Part print with two shaded views. Sizes in mm from the minimum x, y, z corner. A direction names the side the tool comes from. Round coordinates to 2 decimals unless told otherwise and drop trailing zeros. Order: outer loops, then holes, each group sorted by start corner. A loop starts at its lowest first (then second) coordinate and runs counter-clockwise, first axis right, second up. Notation, with made-up numbers: M 9,49.5 L 40,49.5 A28 cw 40,74.5 Z; hole C -6,-6.5 d4. An arc over 180 degrees is marked long. Return JSON: item names as keys, results as strings. Group by question number.
Item 1: Probe line 1 along X through (y, z) = (3.4, 1); line 2 along X through (y, z) = (3.3, 13); line 3 along X through (y, z) = (0.6, 14) (1 decimal). List the from-to ranges inside material, lowest first.
Item 2: Pull direction X, two halves, no side cores. Call the marked faces 1, 2, 3 and 4: pulls with the +X half, pulls with the -X half, needs draft (parallel to the pull), parting line crosses it, or undercut.
Item 3: Slice it at A-A on y = 2.3. Write the cut outline in (x, z), then the cut area to 3 significant figures.
Item 4: Which spindle directions (+Z, -Z, +X, -X, +Y, -Y) get a long thin tool onto all of the face, cutting with end or side? Do the marked faces 5 and 6. Say none if no direction does.
Item 5: Slice it at B-B on x = 8.5. Write the cut outline in (y, z).
Item 6: Slice it at D-D on z = 14. Write the cut outline in (x, y) (1 decimal).
Item 7: Slice it at C-C on z = 18.75. Write the cut outline in (x, y), then the cut area to 3 significant figures.
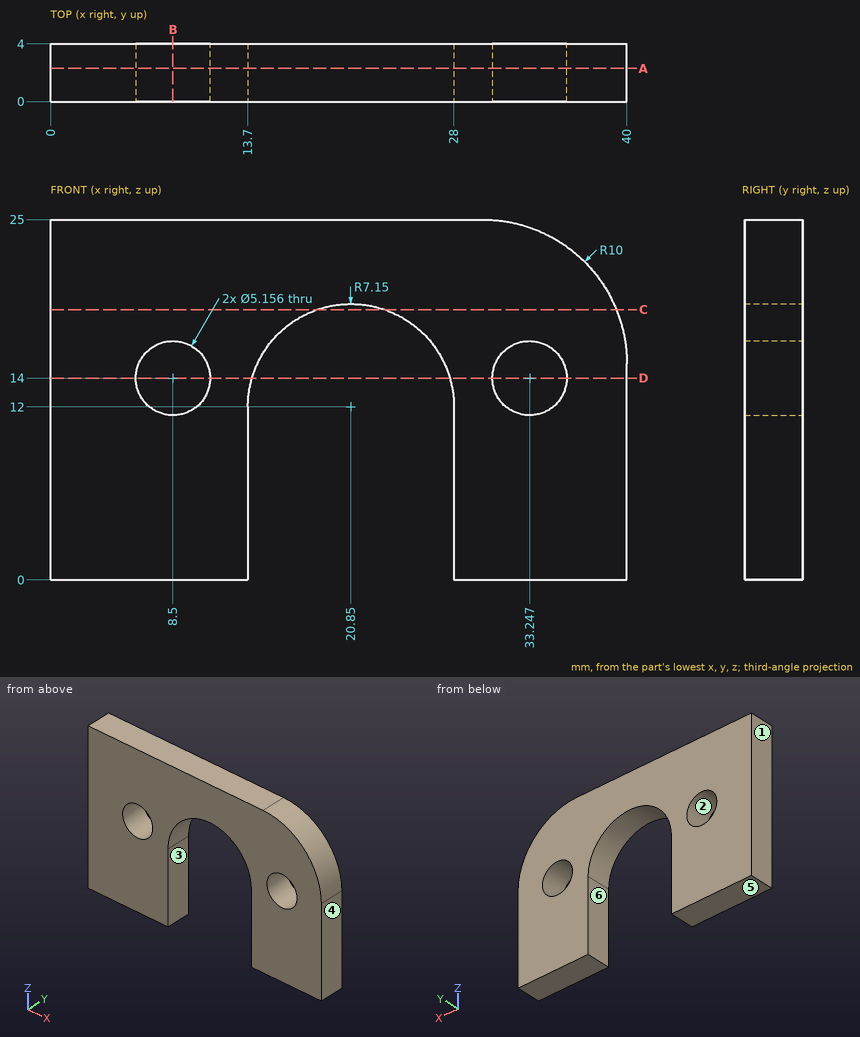
Output values:
{
 "1": {"line 1": "0 to 13.7, 28 to 40", "line 2": "0 to 6.12, 10.88 to 13.77, 27.93 to 30.87, 35.62 to 40", "line 3": "0 to 5.9, 11.1 to 14, 27.7 to 30.7, 35.8 to 40"},
 "2": {"face 1": "pulls with the -X half", "face 2": "undercut", "face 3": "undercut", "face 4": "pulls with the +X half"},
 "3": {"outline": "M 0,0 L 13.7,0 L 13.7,12 A7.15 cw 28,12 L 28,0 L 40,0 L 40,15 A10 ccw 30,25 L 0,25 Z; hole C 8.5,14 d5.16; hole C 33.25,14 d5.16", "area": "685 mm²"},
 "4": {"face 5": "-Z, +X, -X, +Y, -Y", "face 6": "-Z, +Y, -Y"},
 "5": {"outline": "M 0,0 L 4,0 L 4,11.42 L 0,11.42 Z; M 0,16.58 L 4,16.58 L 4,25 L 0,25 Z"},
 "6": {"outline": "M 0,0 L 5.9,0 L 5.9,4 L 0,4 Z; M 11.1,0 L 14,0 L 14,4 L 11.1,4 Z; M 27.7,0 L 30.7,0 L 30.7,4 L 27.7,4 Z; M 35.8,0 L 40,0 L 40,4 L 35.8,4 Z"},
 "7": {"outline": "M 0,0 L 18.49,0 L 18.49,4 L 0,4 Z; M 23.21,0 L 39.27,0 L 39.27,4 L 23.21,4 Z", "area": "138 mm²"}
}
